Could you check a few things on this model? Use its own coordinates, in mm. Face numbers are marked on the shaded views. A direction names the side the tool comes from. Give positions to 0.01 mm unless a question says otherwise; leave off trailing zeros. Order: outer loops, then holes, each group sorted by start corner. A loop starts at its lowest first (then second) coordinate and runs counter-clockwise, first axis right, second up. Notation, with made-up numbers: (-10.75, -13.75) -> (-0.75, -13.75) arc R34 ccw to (-0.75, 16.25) -> close; hole circle Ø9 at (29.25, -1.75). An arc over 180 degrees is marked (long way). Write each question's results on one line, items separated by ' | '.
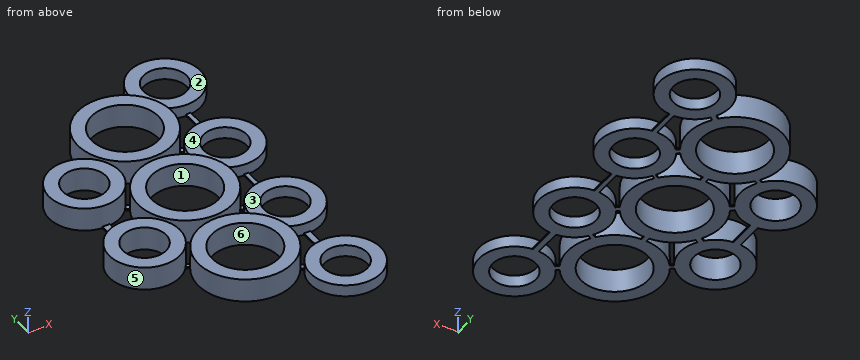
Autodesk Fusion 360 part; units mm, degrees
sketch "Sketch1" plane through (0, 0, 0) normal (0, 0, 1) x (1, 0, 0)
  circle A0 centre (35, 25) radius 4.25
  circle A1 centre (35, 25) radius 6
  circle A2 centre (35, 37.5) radius 6
  circle A3 centre (35, 37.5) radius 4.25
  circle A4 centre (35, 50) radius 6
  circle A5 centre (35, 50) radius 4.25
  circle A6 centre (26, 31.3) radius 4.5
  circle A7 centre (26, 31.3) radius 2.75
  circle A8 centre (26, 43.8) radius 4.5
  circle A9 centre (26, 43.8) radius 2.75
  circle A10 centre (44, 31.3) radius 4.5
  circle A11 centre (44, 31.3) radius 2.75
  circle A12 centre (44, 18.8) radius 2.75
  circle A13 centre (44, 18.8) radius 4.5
  circle A14 centre (44, 56.3) radius 4.5
  circle A15 centre (44, 56.3) radius 2.75
  circle A16 centre (44, 43.8) radius 4.5
  circle A17 centre (44, 43.8) radius 2.75
  line L0 (29.5225, 46.6003) -> (29.8899, 46.8556)
  line L1 (29.8449, 46.1381) -> (30.2075, 46.39)
  line L2 (34.7346, 44.0059) -> (34.7346, 43.4941)
  line L3 (35.433, 44.0156) -> (35.433, 43.2)
  line L4 (29.3463, 40.7913) -> (29.7769, 40.4528)
  line L5 (29.7769, 41.3535) -> (30.1629, 41.05)
  line L6 (29.7769, 34.5472) -> (29.373, 34.2787)
  line L7 (30.1629, 33.95) -> (29.8008, 33.7092)
  line L8 (34.6142, 31.5124) -> (34.6142, 30.9876)
  line L9 (35.2551, 31.5124) -> (35.2551, 30.9946)
  line L10 (29.4191, 28.3743) -> (29.8451, 28.0703)
  line L11 (29.7489, 28.8109) -> (30.1463, 28.5273)
  line L12 (39.7474, 28.6691) -> (40.1698, 28.9378)
  line L13 (40.0613, 28.2223) -> (40.4842, 28.4913)
  line L14 (39.9586, 34.1218) -> (40.3078, 33.8725)
  line L15 (40.3078, 34.7024) -> (40.7354, 34.3972)
  line L16 (40.3078, 22.2024) -> (40.7354, 21.8972)
  line L17 (39.9586, 21.6218) -> (40.3078, 21.3725)
  line L18 (43.6177, 26.8163) -> (43.6177, 23.2837)
  line L19 (44.3823, 26.8163) -> (44.3823, 23.2837)
  line L20 (43.6177, 39.3163) -> (43.6177, 35.7837)
  line L21 (44.1969, 39.3043) -> (44.1969, 35.7957)
  line L22 (40.0129, 41.7137) -> (39.59, 41.3642)
  line L23 (40.2163, 41.3642) -> (39.8367, 41.0505)
  line L24 (39.8151, 46.4203) -> (40.1765, 46.1729)
  line L25 (40.1765, 46.9662) -> (40.5614, 46.7028)
  line L26 (39.5856, 53.8694) -> (39.9958, 54.2466)
  line L27 (39.9958, 53.3229) -> (40.3584, 53.6564)
  line L28 (43.8974, 51.8012) -> (43.8974, 48.2988)
  line L29 (44.5001, 51.8279) -> (44.5001, 48.2721)
  line L30 (25.5335, 39.3242) -> (25.5335, 35.7758)
  line L31 (26.4665, 39.3242) -> (26.4665, 35.7758)
  dimension "d1" = 8.5
  dimension "d2" = 12
  dimension "d5" = 8.5
  dimension "d6" = 12
  dimension "d7" = 8.5
  dimension "d8" = 12
  dimension "d19" = 5.5
  dimension "d20" = 9
  dimension "d21" = 5.5
  dimension "d22" = 9
  dimension "d23" = 5.5
  dimension "d24" = 9
  dimension "d25" = 5.5
  dimension "d26" = 9
  dimension "d27" = 5.5
  dimension "d28" = 9
  dimension "d29" = 5.5
  dimension "d30" = 9
extrude "Extrude1" add sketch "Sketch1" along normal blind 3 contours A1 | A2 | A6 | A8 | A4 makes body 1 at (40.9702, 36.9026, 1) makes body 2 at (30.4776, 30.8519, 1) makes body 3 at (40.9702, 50.5974, 2) makes body 4 at (30.4776, 44.2481, 2) makes body 5 at (40.9702, 24.4026, 1)
extrude "Extrude2" add sketch "Sketch1" along normal blind 1.5 separate body contours A10 | A13 | A16 | A14 makes body 6 at (48.4776, 31.7481, 1) makes body 7 at (48.4776, 43.3519, 0.5) makes body 8 at (48.4776, 18.3519, 0.5) makes body 9 at (48.4776, 56.7481, 1)
extrude "Extrude3" add sketch "Sketch1" along normal blind 0.2 contours A1 A10 L12 L13 | A1 A13 L16 L17 | A1 A2 L8 L9 | A10 A13 L18 L19 | A1 A6 L10 L11 | A2 A10 L14 L15 | A6 A8 L30 L31 | A2 A6 L6 L7 | A10 A16 L20 L21 | A4 A8 L0 L1 | A2 A8 L4 L5 | A2 A16 L22 L23 | A14 A16 L28 L29 | A4 A14 L26 L27 | A2 A4 L2 L3 | A4 A16 L24 L25 bodies 1 2 3 4 5 6 7 8 9
Q1. Suppose I cut it at A-A on z = 0.7. State how many separate pieces and enclosed holes the cut face has, and give its area (3 significant figures).
Here are the results:
separate pieces: 9 | enclosed holes: 9 | area: 408 mm²
Q2. Suppose I cut it at B-B on y = 25. Please give me the cut outline in (x, z), and give its area (3 significant figures).
Here are the results:
outline: (29, 0) -> (30.75, 0) -> (30.75, 3) -> (29, 3) -> close; (39.25, 0) -> (41, 0) -> (41, 3) -> (39.25, 3) -> close; (43.62, 0) -> (44.38, 0) -> (44.38, 0.2) -> (43.62, 0.2) -> close | area: 10.7 mm²
Q3. I need wall thicknesses on line 1 along Y through (x, z) = (35, 1.7); line 2 along Y through (x, z) = (25.75, 2.8); line 3 along Y through (x, z) = (27.5, 0.5). Which ranges of each line are inside material? Lowest first, please.
Here are the results:
line 1: y = 19 to 20.75, 29.25 to 31, 31.5 to 33.25, 41.75 to 43.5, 44 to 45.75, 54.25 to 56 | line 2: y = 26.81 to 28.56, 34.04 to 35.79, 39.31 to 41.06, 46.54 to 48.29 | line 3: y = 27.06 to 29, 33.6 to 35.54, 39.56 to 41.5, 46.1 to 48.04
Q4. I'm going to push flat-ended pins straight in: pin 1 Ø1.5 at (x, z) = (25.5, 1.5) entering from +Y; pin 2 Ø6 at (x, y) = (26, 21) entering from +Z; pin 3 Ø2.5 at (x, y) = (42, 55) entering from +Z; pin 4 Ø0.6 at (x, y) = (44, 38) entering from +Z. Where does each tip first touch, or does it pass through?
Here are the results:
pin 1: stops at y = 48.3 | pin 2: passes through | pin 3: stops at z = 1.5 | pin 4: stops at z = 0.2
Q5. For the marked faces 1, 2 and 3, which set-ups out of +Z, -Z, +X, -X, +Y, -Y let a thin tool reach every point of the face, with its end or its side?
Here are the results:
face 1: +Z, -Z | face 2: +Z, +X, +Y | face 3: +Z, +X
Q6. Thinking about a two-plate mould opening in X: for the marked faces 4, 5 and 6, which applies, +X half, -X half, draft (parallel to the pull), parting line (faces both ways), or undercut?
Here are the results:
face 4: draft | face 5: undercut | face 6: undercut
Q7. Suppose I cut it at C-C on x = 37.25. Please give me the cut outline in (y, z), and give its area (3 significant figures).
Here are the results:
outline: (19.44, 0) -> (21.39, 0) -> (21.39, 3) -> (19.44, 3) -> close; (28.61, 0) -> (30.56, 0) -> (30.56, 3) -> (28.61, 3) -> close; (31.94, 0) -> (33.89, 0) -> (33.89, 3) -> (31.94, 3) -> close; (41.11, 0) -> (43.06, 0) -> (43.06, 3) -> (41.11, 3) -> close; (44.44, 0) -> (46.39, 0) -> (46.39, 3) -> (44.44, 3) -> close; (53.61, 0) -> (55.56, 0) -> (55.56, 3) -> (53.61, 3) -> close | area: 35.2 mm²
